```python
from build123d import *

# Parameters (mm, degrees)
CUT_EXTRUDE3_DEPTH           = 60
CUT_EXTRUDE5_DEPTH           = 2
CUT_EXTRUDE5_DEPTH_BACK      = 30
SKETCH9_R                    = 38
SKETCH9_R_2                  = 23
SKETCH19_W                   = 12
SKETCH19_H                   = 36.5
CUT_REVOLVE2_ANGLE           = 65
CUT_REVOLVE2_OTHER_WAY_ANGLE = 65
SKETCH21_W                   = 3.25
SKETCH21_H                   = 4
BOSS_EXTRUDE3_DEPTH          = 1.35
CIRPATTERN1_COUNT            = 5
CUT_EXTRUDE9_START           = -5
CUT_EXTRUDE9_DEPTH           = 5
SKETCH23_R                   = 10.5
CUT_EXTRUDE10_DEPTH          = 10
SKETCH24_W                   = 15
SKETCH24_H                   = 8
BOSS_EXTRUDE4_DEPTH          = 8
SKETCH26_W                   = 8
SKETCH26_H                   = 5
CUT_EXTRUDE11_DEPTH          = 10
SKETCH27_W                   = 4
SKETCH27_H                   = 5
CUT_EXTRUDE12_DEPTH          = 5
CUT_EXTRUDE14_DEPTH          = 30


# Read off the part's stored shape, not the designer's step: Cut-Extrude9
with BuildPart() as part:
    # Sketch1 → Revolve1 (revolve)
    with BuildSketch(Plane.XY, mode=Mode.PRIVATE) as revolve1_sk:
        with BuildLine():
            Line((0, 63.427876097), (32, 63.427876097))
            ThreePointArc((32, 63.427876097), (37.656854249, 61.084730346), (40, 55.427876097))
            Line((40, 55.427876097), (40, 28.846818009))
            ThreePointArc((40, 28.846818009), (38.792081772, 24.082439968), (35.460140376, 20.469057744))
            Line((35.460140376, 20.469057744), (28.539859624, 15.958818353))
            ThreePointArc((28.539859624, 15.958818353), (25.207918228, 12.345436129), (24, 7.581058088))
            Line((24, 7.581058088), (24, 3.25))
            Line((24, 3.25), (24.35, 3))
            Line((24.35, 3), (24.35, 0))
            Line((24.35, 0), (22.5, 0))
            Line((22.5, 0), (22.5, 12.5))
            ThreePointArc((22.5, 12.5), (22.353553391, 12.853553391), (22, 13))
            Line((22, 13), (0, 13))
            Line((0, 13), (0, 63.427876097))
        make_face()
    revolve(revolve1_sk.sketch.rotate(Axis((0, 0, 0), (0, 1, 0)), 90), axis=Axis((0, 0, 0), (0, 1, 0)))

    # Sketch11 → Cut-Extrude3 (cut)
    with BuildSketch(Plane(origin=(0, 13, 0), x_dir=(-1, 0, 0), z_dir=(0, -1, 0))):
        with BuildLine():
            Line((-21, 0), (21, 0))
            ThreePointArc((21, 0), (0, 21), (-21, 0))
        make_face()
    extrude(amount=-CUT_EXTRUDE3_DEPTH, mode=Mode.SUBTRACT)

    # Sketch9 → Cut-Extrude5 (cut, two sides: drawn at the far end of the back side and taken through both)
    with BuildSketch(Plane(origin=(0, 55.427876097, 0), x_dir=(1, 0, 0), z_dir=(0, 1, 0)).offset(-CUT_EXTRUDE5_DEPTH_BACK)):
        with Locations(Location((0, 0, 0), (0, 0, 270))):
            Circle(SKETCH9_R)
        with Locations(Location((0, 0, 0), (0, 0, 270))):
            Circle(SKETCH9_R_2, mode=Mode.SUBTRACT)
    extrude(amount=CUT_EXTRUDE5_DEPTH + CUT_EXTRUDE5_DEPTH_BACK, mode=Mode.SUBTRACT)

    # Sketch19 → Cut-Revolve2 (revolve, cut)
    with BuildSketch(Plane(origin=(0, 0, 0), x_dir=(0, 0, -1), z_dir=(1, 0, 0))):
        with Locations((-41.064715832, 37.177876097)):
            Rectangle(SKETCH19_W, SKETCH19_H)
    revolve(axis=Axis((0, 0, 0), (0, 1, 0)), revolution_arc=CUT_REVOLVE2_ANGLE, mode=Mode.SUBTRACT)

    # Sketch19 → Cut-Revolve2 other way (revolve, cut)
    with BuildSketch(Plane(origin=(0, 0, 0), x_dir=(0, 0, -1), z_dir=(1, 0, 0))):
        with Locations((-41.064715832, 37.177876097)):
            Rectangle(SKETCH19_W, SKETCH19_H)
    revolve(axis=Axis((0, 0, 0), (0, -1, 0)), revolution_arc=CUT_REVOLVE2_OTHER_WAY_ANGLE, mode=Mode.SUBTRACT)

    # Sketch21 → Boss-Extrude3 (add)
    with BuildSketch(Plane(origin=(0, 0, 22.5), x_dir=(-1, 0, 0), z_dir=(0, 0, -1))):
        with Locations((0, 2)):
            Rectangle(SKETCH21_W, SKETCH21_H)
    boss_extrude3 = extrude(amount=BOSS_EXTRUDE3_DEPTH)

    # CirPattern1: Boss-Extrude3 ×5 about axis
    cirpattern1_axis = Axis((0, 0, 0), (0, 1, 0))
    for i in range(1, CIRPATTERN1_COUNT):
        add(boss_extrude3.rotate(cirpattern1_axis, i * 360 / CIRPATTERN1_COUNT))

    # Cut-Extrude9 outline → Cut-Extrude9 (cut)
    with BuildSketch(Plane(origin=(0, 63.427876097, 0), x_dir=(1, 0, 0), z_dir=(0, 1, 0)).offset(CUT_EXTRUDE9_START)):
        with BuildLine():
            ThreePointArc((40, 0), (0, 40), (-40, 0))
            Line((-40, 0), (-21, 0))
            ThreePointArc((-21, 0), (0, 21), (21, 0))
            Line((21, 0), (40, 0))
        make_face()
    extrude(amount=CUT_EXTRUDE9_DEPTH, mode=Mode.SUBTRACT)

    # Sketch23 → Cut-Extrude10 (cut)
    with BuildSketch(Plane(origin=(0, 0, -40), x_dir=(-1, 0, 0), z_dir=(0, 0, -1))):
        with Locations((0, 42.137876097)):
            Circle(SKETCH23_R)
    extrude(amount=-CUT_EXTRUDE10_DEPTH, mode=Mode.SUBTRACT)

    # Sketch24 → Boss-Extrude4 (add)
    with BuildSketch(Plane(origin=(0, 58.427876097, 0), x_dir=(1, 0, 0), z_dir=(0, 1, 0))):
        with Locations((0, 30)):
            Rectangle(SKETCH24_W, SKETCH24_H)
    extrude(amount=-BOSS_EXTRUDE4_DEPTH)

    # Sketch26 → Cut-Extrude11 (cut)
    with BuildSketch(Plane(origin=(0, 58.427876097, 0), x_dir=(1, 0, 0), z_dir=(0, 1, 0))):
        with Locations((0, 30)):
            Rectangle(SKETCH26_W, SKETCH26_H)
    extrude(amount=-CUT_EXTRUDE11_DEPTH, mode=Mode.SUBTRACT)

    # Sketch27 → Cut-Extrude12 (cut)
    with BuildSketch(Plane(origin=(7.5, 0, 0), x_dir=(0, 0, -1), z_dir=(1, 0, 0))):
        with Locations((30, 53.927876097)):
            Rectangle(SKETCH27_W, SKETCH27_H)
    extrude(amount=-CUT_EXTRUDE12_DEPTH, mode=Mode.SUBTRACT)

    # Sketch28 → Cut-Extrude14 (cut)
    with BuildSketch(Plane(origin=(0, 55.427876097, 0), x_dir=(1, 0, 0), z_dir=(0, 1, 0))):
        with BuildLine():
            Line((-22.912878475, -2), (22.912878475, -2))
            ThreePointArc((22.912878475, -2), (0, -23), (-22.912878475, -2))
        make_face()
    extrude(amount=-CUT_EXTRUDE14_DEPTH, mode=Mode.SUBTRACT)


solid = part.part
```
Could you check a few things on this model? Use its own coordinates, in mm. A direction names the side the tool comes from. Coordinates: 2 decimals unless noted, no trailing zeros. Write each loop counter-clockwise with the first axis right and the second up, starting at its lowest first coordinate (ties: lowest second). Pieces come first, ordered by that corner, then holes. Notation, with made-up numbers: (-6, -4.5) -> (35, -4.5) arc R29 cw to (35, 20.5) -> close; hole circle Ø9 at (61, 50.25). An arc over 180 degrees is marked (long way). One line per question, with ' | ' between items. Start each with the question number.
1. If we section it at B-B (y = 5.5): Please give me the cut outline in (x, z), and give its area (3 significant figures).
2. If we section it at D-D (y = 33): Please give me the cut outline in (x, z).
3. Please list where these lines run through material, in increasing order: line 1 along Z through (x, y) = (0, 51); line 2 along X through (y, z) = (4, 0); line 3 along Z through (x, y) = (0, 36).
4. Will these pins go through, and if not, where does the flat tip stop? P1, Ø2, axis at y = 34, z = -22, coming from the +X side; P2, Ø6, axis at x = -25.5, y = 40, coming from the +Z side; P3, Ø5.5, axis at y = 56, z = -29, coming from the -X side.
5. If we section it at A-A (y = 49): Please give me the cut outline in (x, z).
6. For faces 4 (the face through (0, 2, 21.15)), 5 (the face through (0, 41, 2)), 6 (the face through (0, 35, -21)), 7 (the face through (1.011, 41.204, -22.978)), which set-ups out of +Z, -Z, +X, -X, +Y, -Y let a thin tool reach every point of the face, with its end or its side?
7. If we section it at C-C (x = 0): Count the separate pieces of the cut face and the enclosed holes in it, and give its area (3 significant figures).
8. Thinking about a two-plate mould opening in Z: for faces 1 (the face through (13, 0, -18)), 2 (the face through (-35.04, 38.07, 16.34)), 3 (the face through (12.413, 2.028, -17.124)), which applies, pulls with the +Z half, pulls with the -Z half, needs draft (parallel to the pull), parting line crosses it, or undercut?
Return value:
1) outline: circle Ø48 at (0, 0); hole circle Ø45 at (0, 0) | area: 219 mm²
2) outline: (-36.25, 16.9) arc R40 ccw to (-5.17, -39.66) -> (-5.17, -37.65) arc R38 cw to (-34.44, 16.06) -> close; (-22.91, 2) arc R23 ccw (long way) to (22.91, 2) -> close; (5.17, -39.66) arc R40 ccw to (36.25, 16.9) -> (34.44, 16.06) arc R38 cw to (5.17, -37.65) -> close; hole (-21, 0) arc R21 ccw to (21, 0) -> close
3) line 1: z = -34 to -32.5, -27.5 to -26, -23 to -21, 0 to 2 | line 2: x = -24 to -22.5, 22.5 to 24 | line 3: z = -23 to -21, 0 to 2
4) P1: stops at x = 34.04 | P2: stops at z = 2 | P3: stops at x = -30.16
5) outline: (-36.25, 16.9) arc R40 ccw to (-7.95, -39.2) -> (-7.95, -37.16) arc R38 cw to (-34.44, 16.06) -> close; (-22.91, 2) arc R23 ccw (long way) to (22.91, 2) -> close; (7.95, -39.2) arc R40 ccw to (36.25, 16.9) -> (34.44, 16.06) arc R38 cw to (7.95, -37.16) -> close; hole (-21, 0) arc R21 ccw to (21, 0) -> close
6) face 4: -Y | face 5: +Z | face 6: +Y, -Y | face 7: none
7) separate pieces: 3 | enclosed holes: 0 | area: 1,060 mm²
8) face 1: needs draft | face 2: pulls with the +Z half | face 3: undercut
